Geometry: final body of the model. Coordinates: model frame, mm. A direction names the side the tool comes from. Give positions to 0.01 mm unless a question says otherwise; leave off trailing zeros. Loops run counter-clockwise (first coordinate to the right, second up) from the corner with the lowest first, then second, coordinate; pieces in that order, holes last.
```python
from build123d import *

# Parameters (mm, degrees)
F0_R     = 22.5
F0_R_2   = 17.5
F1_DEPTH = 48
F2_W     = 60
F2_H     = 60
F2_R     = 22.5
F2_R_2   = 17.5
F3_DEPTH = 32
F4_W     = 30
F4_H     = 15
F5_DEPTH = 60.001
F7_DEPTH = 48


with BuildPart() as f1:
    # F0 (on Front) → F1 (new body)
    with BuildSketch(Plane.XZ):
        Circle(F0_R)
        Circle(F0_R_2, mode=Mode.SUBTRACT)
    extrude(amount=F1_DEPTH)

    # F2 (on face) → F3 (join)
    with BuildSketch(Plane(origin=(0, 0, 0), x_dir=(-1, 0, 0), z_dir=(0, 1, 0))):
        Rectangle(F2_W, F2_H)
        Circle(F2_R, mode=Mode.SUBTRACT)
        Circle(F2_R)
        Circle(F2_R_2, mode=Mode.SUBTRACT)
    extrude(amount=F3_DEPTH)

    # F4 (on face) → F5 (cut, through all)
    with BuildSketch(Plane(origin=(0, 0, -30), x_dir=(1, 0, 0), z_dir=(0, 0, -1))):
        with Locations((0, -24.5)):
            Rectangle(F4_W, F4_H)
    extrude(amount=-F5_DEPTH, mode=Mode.SUBTRACT)

    # F6 (on face) → F7 (cut, through all)
    with BuildSketch(Plane.XZ.offset(48)):
        with BuildLine():
            ThreePointArc((-21.2132034356, 7.5), (-22.5, 0), (-21.2132034356, -7.5))
            Line((-21.2132034356, -7.5), (-15.8113883008, -7.5))
            ThreePointArc((-15.8113883008, -7.5), (-17.5, 0), (-15.8113883008, 7.5))
            Line((-15.8113883008, 7.5), (-21.2132034356, 7.5))
        make_face()
        with BuildLine():
            Line((15.8113883008, -7.5), (21.2132034356, -7.5))
            ThreePointArc((21.2132034356, -7.5), (22.1759675922, -3.8047945213), (22.5, 0))
            ThreePointArc((22.5, 0), (22.1759675922, 3.8047945213), (21.2132034356, 7.5))
            Line((21.2132034356, 7.5), (15.8113883008, 7.5))
            ThreePointArc((15.8113883008, 7.5), (17.0726286093, 3.843872054), (17.5, 0))
            ThreePointArc((17.5, 0), (17.0726286093, -3.843872054), (15.8113883008, -7.5))
        make_face()
    extrude(amount=-F7_DEPTH, mode=Mode.SUBTRACT)


solid = f1.part
```
Q1. Mould query, pull axis Z, two halves, no side actions, for faces 4 (the face through (0.388, -23.664, 22.497)), 5 (the face through (0, 17, -22)), 6 (the face through (-18, -24, 7.5)). Classes: +Z half, -Z half, draft (parallel to the pull), parting line (faces both ways), or undercut.
Q2. Section query D-D, the plane y = 4. Return loops of the section in (x, z), and give its area (3 significant figures).
Q3. Material intervals for probe 1 along Z at (x, y) = (0, 13); probe 2 along Z at (x, y) = (-16, -12.5); probe 3 along Y at (x, z) = (0, -20.5), sorted ascending.
Q4. Pin query (flat end, axial travel): pin 1 Ø10.5 at (x, z) = (-6, -15) entering from +Y; pin 2 Ø6 at (x, y) = (-20, -19) entering from -Z; pin 3 Ø10 at (x, y) = (2.5, -24.5) entering from -Z. Return the tip coordinate at first contact, or that it passes through.
Q5. Reachability of faces 1 (the face through (19, -24, 7.5)), 2 (the face through (-0.388, -23.664, -22.497)), 3 (the face through (-15, 25, -20)) from +Z, -Z, +X, -X, +Y, -Y: full face, straight path, thin tool, end or side. Return the list, or none.
Q6. Section query B-B, the plane y = -21. Return loops of the section in (x, z), and give its area (3 significant figures).
Q7. Section query C-C, the plane z = 0. Return loops of the section in (x, y).
Q8. Section query A-A, the plane x = -7.5. Return loops of the section in (y, z).
Resolved:
1. face 4: +Z half
1. face 5: draft
1. face 6: undercut
2. outline: (-30, -30) - (30, -30) - (30, 30) - (-30, 30) - close; hole circle Ø35 at (0, 0)
2. area: 2,640 mm2
3. probe 1: z = -30 to -17.5, 17.5 to 30
3. probe 2: z = -15.82 to -7.5, 7.5 to 15.82
3. probe 3: y = -48 to 17
4. pin 1: stops at y = 17
4. pin 2: stops at z = -14.74
4. pin 3: stops at z = -22.5
5. face 1: +X, -X, -Y
5. face 2: -Z, -Y
5. face 3: +Z, -Z, +Y
6. outline: (-21.21, -7.5) arc R22.5 ccw to (21.21, -7.5) - (15.81, -7.5) arc R17.5 cw to (-15.81, -7.5) - close; (-21.21, 7.5) - (-15.81, 7.5) arc R17.5 cw to (15.81, 7.5) - (21.21, 7.5) arc R22.5 ccw to start
6. area: 474 mm2
7. outline: (-30, 0) - (-17.5, 0) - (-17.5, 32) - (-30, 32) - close; (17.5, 0) - (30, 0) - (30, 32) - (17.5, 32) - close
8. outline: (-48, -21.21) - (0, -21.21) - (0, -30) - (17, -30) - (17, -15.81) - (-48, -15.81) - close; (-48, 15.81) - (17, 15.81) - (17, 30) - (0, 30) - (0, 21.21) - (-48, 21.21) - close
